Autodesk Fusion 360 part; units mm, degrees
ref_plane "WorkPlane1" through (0, 0, 40) normal (0, 0, 1) x (1, 0, 0)
sketch "Sketch1" plane through (0, 0, 40) normal (0, 0, 1) x (1, 0, 0)
  line L0 (-10, 50) -> (75, 50)
  line L1 (75, 50) -> (75, -10)
  line L2 (75, -10) -> (-10, -10)
  line L3 (-10, -10) -> (-10, 50)
extrude "Extrude1" add sketch "Sketch1" along normal blind 10
sketch "Sketch2" plane through (0, 0, 50) normal (0, 0, 1) x (-1, 0, 0)
  line L0 (10, 10) -> (-75, 10)
  line L1 (-75, 10) -> (-75, -50)
  line L2 (-75, -50) -> (10, -50)
  line L3 (10, -50) -> (10, 10)
  circle A0 centre (-10, 5) radius 2.5
  circle A1 centre (-55, 5) radius 2.5
  circle A2 centre (-55, -45) radius 2.5
  circle A3 centre (-10, -45) radius 2.5
  dimension "d11" = 5
  dimension "d12" = 5
  dimension "d13" = 5
  dimension "d14" = 5
extrude "Extrude2" cut sketch "Sketch2" against normal blind 10 contours A0 | A1 | A2 | A3
Here's how the part is built. I have some questions about the finished solid (model axes, mm). Coordinates: 2 decimals unless noted, no trailing zeros. Loops run counter-clockwise (first coordinate to the right, second up) from the corner with the lowest first, then second, coordinate; pieces in that order, holes last. Notation, with made-up numbers: (5.25, 74) -> (63.25, 74) arc R34 ccw to (63.25, 105) -> close; hole circle Ø2 at (-34.75, 64.5). An arc over 180 degrees is marked (long way). Return JSON: item names as keys, results as strings.
1) If we section it at B-B, the plane x = 55: Write out the boundary of the cut face in (y, z), then the cut area to 3 significant figures.
Results below:
{"outline": "(-10, 40) -> (-7.5, 40) -> (-7.5, 50) -> (-10, 50) -> close; (-2.5, 40) -> (42.5, 40) -> (42.5, 50) -> (-2.5, 50) -> close; (47.5, 40) -> (50, 40) -> (50, 50) -> (47.5, 50) -> close", "area": "500 mm²"}
2) I need wall thicknesses on line 1 (Y direction, x = 10, z = 47.5); line 2 (X direction, y = -5, z = 42.75); line 3 (Y direction, x = 11, z = 49). Which ranges of each line are inside material? Lowest first, please. Write a range as from..to.
Results below:
{"line 1": "-10..-7.5, -2.5..42.5, 47.5..50", "line 2": "-10..7.5, 12.5..52.5, 57.5..75", "line 3": "-10..-7.29, -2.71..42.71, 47.29..50"}
3) Will this pin go through, and if not, where does the flat tip stop? pin 1 (3 mm diameter, centred on x = 55, y = 45, fed in from +Z).
Results below:
{"pin 1": "through"}
4) If we section it at C-C, the plane z = 43.5: Write out the boundary of the cut face in (x, y).
Results below:
{"outline": "(-10, -10) -> (75, -10) -> (75, 50) -> (-10, 50) -> close; hole circle Ø5 at (10, -5); hole circle Ø5 at (10, 45); hole circle Ø5 at (55, -5); hole circle Ø5 at (55, 45)"}
5) Thinking about a two-plate mould opening in X: for faces 1 (the face through (75, 20, 45)), 2 (the face through (10.54, 47.44, 45.07)), 3 (the face through (32, 20, 40)), which applies, +X half, -X half, draft (parallel to the pull), parting line (faces both ways), or undercut?
Results below:
{"face 1": "+X half", "face 2": "undercut", "face 3": "draft"}
6) If we section it at A-A, the plane y = 45: Write out the boundary of the cut face in (x, z), then the cut area to 3 significant figures.
Results below:
{"outline": "(-10, 40) -> (7.5, 40) -> (7.5, 50) -> (-10, 50) -> close; (12.5, 40) -> (52.5, 40) -> (52.5, 50) -> (12.5, 50) -> close; (57.5, 40) -> (75, 40) -> (75, 50) -> (57.5, 50) -> close", "area": "750 mm²"}
